```python
from build123d import *

# Parameters (mm, degrees)
F0_R     = 4.6188021535
F0_R_2   = 2.5
F1_DEPTH = 1.6
F2_R     = 0.6
F3_R     = 7.5
F4_DEPTH = 3.2010001


with BuildPart() as f1:
    # F0 (on Top) → F1 (new body, symmetric)
    with BuildSketch(Plane.XY):
        Circle(F0_R)
        Circle(F0_R_2, mode=Mode.SUBTRACT)
    extrude(amount=F1_DEPTH, both=True)

    # F2
    f2_edges = [f1.edges().sort_by_distance(p)[0] for p in [
        (-4.618802, 0, 1.6),
        (-4.618802, 0, -1.6),
    ]]
    fillet(f2_edges, radius=F2_R)

    # F3 (on face) → F4 (cut, through all)
    with BuildSketch(Plane.XY.offset(1.6)):
        Circle(F3_R)
        Polygon((-2.3094010768, -4), (-4.6188021535, 0), (-2.3094010768, 4), (2.3094010768, 4), (4.6188021535, 0), (2.3094010768, -4), align=None, mode=Mode.SUBTRACT)
    extrude(amount=-F4_DEPTH, mode=Mode.SUBTRACT)


solid = f1.part
```
Could you check a few things on this model? Use its own coordinates, in mm. Coordinates: 2 decimals unless noted, no trailing zeros. Write each loop counter-clockwise with the first axis right and the second up, starting at its lowest first coordinate (ties: lowest second). Pieces come first, ordered by that corner, then holes. Notation, with made-up numbers: (78, 41) - (90, 41) arc R19 ccw to (90, 73) - close; hole circle Ø8 at (-36, 3.25). An arc over 180 degrees is marked (long way). Use a Markdown table: item, result.
Q1. Imagine slicing it at B-B (x = 0). List the corners of the cut face in (y, z) for me, and give its area (3 significant figures).
Geometry check:
| item | result |
|---|---|
| outline | (-4, -1.6) - (-2.5, -1.6) - (-2.5, 1.6) - (-4, 1.6) - close; (2.5, -1.6) - (4, -1.6) - (4, 1.6) - (2.5, 1.6) - close |
| area | 9.60 mm2 |
Q2. Please list where these lines run through material, in increasing order: L1, parallel to Y at x = 0, z = -0.2; L2, parallel to Z at x = 4, y = 0.75; L3, parallel to Y at x = -1, z = -0.6.
Geometry check:
| item | result |
|---|---|
| L1 | y = -4 to -2.5, 2.5 to 4 |
| L2 | z = -1.6 to 1.6 |
| L3 | y = -4 to -2.29, 2.29 to 4 |
Q3. Thinking about a two-plate mould opening in Y: for faces 1 (the cylindrical face through (-0.54, -2.44, -0.02)), 2 (the flat face through (3.448, 2.028, 0.022)), 3 (the flat face through (-3.448, -2.028, 0.022)), which applies, +Y half, -Y half, draft (parallel to the pull), parting line (faces both ways), or undercut?
Geometry check:
| item | result |
|---|---|
| face 1 | undercut |
| face 2 | +Y half |
| face 3 | -Y half |
Q4. Imagine slicing it at C-C (y = -2). List the corners of the cut face in (x, z) for me, and give its area (3 significant figures).
Geometry check:
| item | result |
|---|---|
| outline | (-3.46, -1.6) - (-1.5, -1.6) - (-1.5, 1.6) - (-3.46, 1.6) - close; (1.5, -1.6) - (3.46, -1.6) - (3.46, 1.6) - (1.5, 1.6) - close |
| area | 12.6 mm2 |
Q5. I'm going to push flat-ended pins straight in: pin 1 Ø1 at (x, z) = (-3, 0.5) entering from -Y; pin 2 Ø1.5 at (x, z) = (-3.5, -1.5) entering from -Y; pin 3 Ø4.5 at (x, y) = (0, 0) entering from -Z; pin 4 Ø4 at (x, y) = (-1.5, 0) entering from +Z. Where does each tip first touch, or does it pass through?
Geometry check:
| item | result |
|---|---|
| pin 1 | stops at y = -3.67 |
| pin 2 | stops at y = -3.24 |
| pin 3 | passes through |
| pin 4 | stops at z = 1.6 |
Q6. Imagine slicing it at A-A (z = 0.1). List the corners of the cut face in (x, y) for me, and give its area (3 significant figures).
Geometry check:
| item | result |
|---|---|
| outline | (-4.62, 0) - (-2.31, -4) - (2.31, -4) - (4.62, 0) - (2.31, 4) - (-2.31, 4) - close; hole circle Ø5 at (0, 0) |
| area | 35.8 mm2 |
